from build123d import *

# Parameters (mm, degrees)
EXTRUDE_1_DEPTH     = 20
SKETCH_2_W          = 4
SKETCH_2_H          = 30
EXTRUDE_2_DEPTH     = 100
CUT_EXTRUDE_1_DEPTH = 100
SKETCH_4_W          = 50
SKETCH_4_H          = 10
EXTRUDE_3_DEPTH     = 50


with BuildPart() as part:
    # 草图1 → 凸台-拉伸1 (new body)
    with BuildSketch(Plane(origin=(0, 0, 0), x_dir=(0, 0, -1), z_dir=(1, 0, 0))):
        with BuildLine():
            Line((-25, 5), (25, 5))
            Line((25, 5), (25, -5))
            Line((25, -5), (25, -11.698777218))
            ThreePointArc((25, -11.698777218), (37.410642162, -21.801835726), (46, -35.304382227))
            Line((46, -35.304382227), (46, -25.083062159))
            Line((46, -25.083062159), (50, -25.083062159))
            Line((50, -25.083062159), (50, -85.083062159))
            Line((50, -85.083062159), (46, -85.083062159))
            Line((46, -85.083062159), (46, -55.083062159))
            ThreePointArc((46, -55.083062159), (0, -9.083062159), (-46, -55.083062159))
            Line((-46, -55.083062159), (-46, -85.083062159))
            Line((-46, -85.083062159), (-50, -85.083062159))
            Line((-50, -85.083062159), (-50, -25.083062159))
            Line((-50, -25.083062159), (-46, -25.083062159))
            Line((-46, -25.083062159), (-46, -35.304382227))
            ThreePointArc((-46, -35.304382227), (-37.410642162, -21.801835726), (-25, -11.698777218))
            Line((-25, -11.698777218), (-25, -5))
            Line((-25, -5), (-25, 5))
        make_face()
    extrude(amount=EXTRUDE_1_DEPTH)

    # 草图2 → 凸台-拉伸2 (add)
    with BuildSketch(Plane(origin=(20, 0, 0), x_dir=(0, 0, -1), z_dir=(1, 0, 0))):
        with Locations((-48, -70.083062159)):
            Rectangle(SKETCH_2_W, SKETCH_2_H)
        with Locations((48, -70.083062159)):
            Rectangle(SKETCH_2_W, SKETCH_2_H)
    extrude(amount=EXTRUDE_2_DEPTH)

    # 草图3 → 切除-拉伸1 (cut)
    with BuildSketch(Plane.XY.offset(50)):
        with BuildLine():
            Line((105, -55.083062159), (132.360099234, -55.083062159))
            Line((132.360099234, -55.083062159), (132.360099234, -85.083062159))
            Line((132.360099234, -85.083062159), (105, -85.083062159))
            ThreePointArc((105, -85.083062159), (120, -70.083062159), (105, -55.083062159))
        make_face()
    extrude(amount=-CUT_EXTRUDE_1_DEPTH, mode=Mode.SUBTRACT)

    # 草图4 → 凸台-拉伸3 (add)
    with BuildSketch(Plane.ZY):
        Rectangle(SKETCH_4_W, SKETCH_4_H)
    extrude(amount=EXTRUDE_3_DEPTH)


solid = part.part
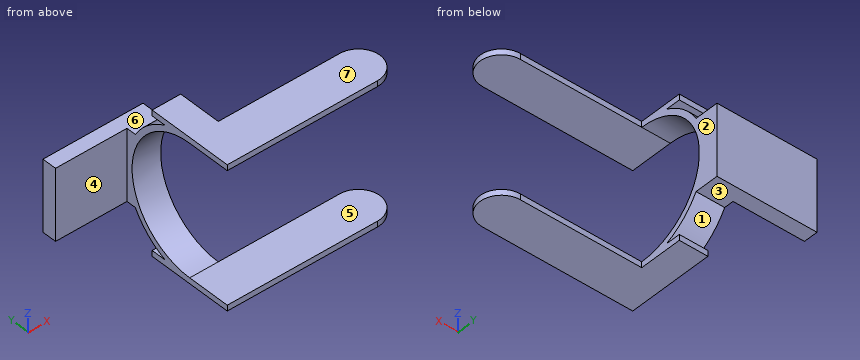
Can you work these out from the model? Positions are in its coordinate system, mm. Face numbers are marked on the shaded views. A direction names the side the tool comes from. Give positions to 0.01 mm unless a question says otherwise; leave off trailing zeros. Loops run counter-clockwise (first coordinate to the right, second up) from the corner with the lowest first, then second, coordinate; pieces in that order, holes last. Notation, with made-up numbers: (78.25, 6.5) - (117.25, 6.5) arc R27 ccw to (117.25, 35.5) - close; hole circle Ø9 at (34, -30). An arc over 180 degrees is marked (long way). Answer as a JSON object with one key per item and string values.
Q1. If we mould it in two halves opening along Z, with no side actions, what happens to the marked faces 1, 2 and 3? For each: pulls with the +Z half, pulls with the -Z half, needs draft (parallel to the pull), parting line crosses it, or undercut.
Geometry says:
{"face 1": "undercut", "face 2": "needs draft", "face 3": "pulls with the -Z half"}
Q2. Imagine slicing it at C-C on z = 0. Write out the boundary of the cut face in (x, y), plus the area to 3 significant figures.
Geometry says:
{"outline": "(-50, -5) - (0, -5) - (0, -9.08) - (20, -9.08) - (20, 5) - (-50, 5) - close", "area": "782 mm²"}
Q3. If I drill on L1, parallel to Z at x = 14, y = -77; L2, parallel to X at y = -26, z = 37.5; L3, parallel to X at y = -3, z = 13.5, over which ranges is the centre line in solid material (lowest first)?
Geometry says:
{"L1": "-50 to -46, 46 to 50", "L2": "0 to 20", "L3": "-50 to 20"}
Q4. Imagine slicing it at D-D on z = -21. Write out the boundary of the cut face in (x, y), plus the area to 3 significant figures.
Geometry says:
{"outline": "(-50, -5) - (0, -5) - (0, -14.16) - (20, -14.16) - (20, 5) - (-50, 5) - close", "area": "883 mm²"}
Q5. Which directions (+Z, -Z, +X, -X, +Y, -Y) give clear straight access to the entire face, cutting with the end or side of a thin tool? Please do the marked faces 4, 5, 6 and 7.
Geometry says:
{"face 4": "+Z, -Z, -X, -Y", "face 5": "+X, -X, -Y", "face 6": "+Z, +X, -X, +Y", "face 7": "+Z, +X, -X, +Y, -Y"}
Q6. Imagine slicing it at B-B on y = -57. Write out the boundary of the cut face in (x, z), plus the area to 3 significant figures.
Geometry says:
{"outline": "(0, -50) - (112.34, -50) - (112.34, -46) - (0, -46) - close; (0, 46) - (112.34, 46) - (112.34, 50) - (0, 50) - close", "area": "899 mm²"}
Q7. Imagine slicing it at A-A on x = 69. Write out the boundary of the cut face in (y, z).
Geometry says:
{"outline": "(-85.08, -50) - (-55.08, -50) - (-55.08, -46) - (-85.08, -46) - close; (-85.08, 46) - (-55.08, 46) - (-55.08, 50) - (-85.08, 50) - close"}
Q8. Will these pins go through, and if not, where does the flat tip stop? P1, Ø18.5, axis at x = -7.5, y = 0, coming from the -Z side; P2, Ø1.2, axis at x = 81.5, z = -48, coming from the +Y side; P3, Ø2, axis at x = -14, z = -19, coming from the -Y side.
Geometry says:
{"P1": "z = -25", "P2": "y = -55.08", "P3": "y = -5"}
